```python
from build123d import *

# Parameters (mm, degrees)
F0_W      = 117
F0_H      = 85
F1_DEPTH  = 3.5
F2_R      = 4.5
F3_DEPTH  = 25
F4_R      = 30
F5_DEPTH  = 1
F7_R      = 25
F8_DEPTH  = 2
F9_R      = 20
F10_DEPTH = 2
F11_R     = 1
F12_R     = 10
F13_DEPTH = 25


# Not quite as in the source:
# - a fillet or chamfer that OpenCascade refuses, or shapes differently, is made with other operations: its cross-section is extruded or revolved along the edge and cut away or added


with BuildPart() as f1:
    # F0 (on Top) → F1 (new body)
    with BuildSketch(Plane.XY):
        Rectangle(F0_W, F0_H)
    extrude(amount=F1_DEPTH)

    # F2 (on face) → F3 (cut)
    with BuildSketch(Plane.XY.offset(3.5)):
        with Locations((40, 30)):
            Circle(F2_R)
        with Locations((-40, 30)):
            Circle(F2_R)
        with Locations((-40, -30)):
            Circle(F2_R)
        with Locations((40, -30)):
            Circle(F2_R)
    extrude(amount=-F3_DEPTH, mode=Mode.SUBTRACT)

    # F4 (on face) → F5 (join)
    with BuildSketch(Plane.XY.offset(3.5)):
        Circle(F4_R)
    extrude(amount=F5_DEPTH)

    # F6: fillet of radius 5 on 1 edges, made by hand

    # F6_s1 → F6_t2 (revolve, cut)
    with BuildSketch(Plane.XZ):
        with BuildLine():
            ThreePointArc((30, 3.5), (28.5811388301, 4.2434164903), (27, 4.5))
            Line((27, 4.5), (30, 4.5))
            Line((30, 4.5), (30, 3.5))
        make_face()
    revolve(axis=Axis((0, 0, 4.5), (0, 0, 1)), mode=Mode.SUBTRACT)

    # F7 (on face) → F8 (cut)
    with BuildSketch(Plane.XY.offset(4.5)):
        Circle(F7_R)
    extrude(amount=-F8_DEPTH, mode=Mode.SUBTRACT)

    # F9 (on face) → F10 (join)
    with BuildSketch(Plane.XY.offset(2.5)):
        Circle(F9_R)
    extrude(amount=F10_DEPTH)

    # F11
    f11_edges = [f1.edges().sort_by_distance(p)[0] for p in [
        (-20, 0, 4.5),
    ]]
    fillet(f11_edges, radius=F11_R)

    # F12 (on face) → F13 (cut)
    with BuildSketch(Plane.XY.offset(4.5)):
        Circle(F12_R)
    extrude(amount=-F13_DEPTH, mode=Mode.SUBTRACT)


solid = f1.part
```
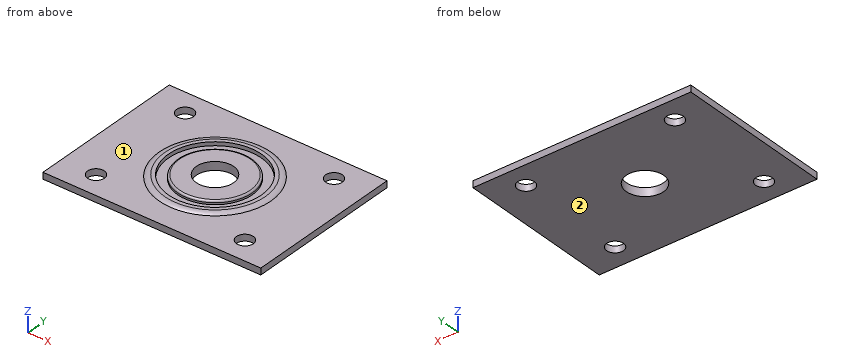
Geometry: final body of the model. Coordinates: model frame, mm. Face numbers are marked on the shaded views. Round coordinates to 2 decimals unless told otherwise and drop trailing zeros. Order: outer loops, then holes, each group sorted by start corner. A loop starts at its lowest first (then second) coordinate and runs counter-clockwise, first axis right, second up. Notation, with made-up numbers: (-4, 55.25) -> (30, 55.25) arc R26 cw to (30, 85.25) -> close; hole circle Ø7 at (-33, 56). An arc over 180 degrees is marked (long way). Use CSV: the item, a comma, the result in double quotes. Start each with the question number.
1) Section B-B (y = 0). Return the cut outline in (x, z), and give its area (3 significant figures).
2) Section D-D (x = 38.5). Return the cut outline in (y, z).
3) Section C-C (z = 1.25). Return the cut outline in (x, y), and give its area (3 significant figures).
4) First-contact query: pin 1 Ø3 at (x, y) = (35.5, 17.5) entering from +Z; pin 2 Ø2 at (x, y) = (-13.5, -18) entering from +Z. Flat tips, straight axial feed; report the tip coordinate or a pass-through.
5) Section A-A (x = -40). Return the cut outline in (y, z).
6) Material intervals for line 1 along Y through (x, z) = (40, 2.25); line 2 along X through (y, z) = (11, 3.45); line 3 along Y through (x, z) = (0, 3.85), sorted ascending. Write a range as from..to.
7) Draft query along Z for the marked faces 1 and 2. Return one class per face: +Z half, -Z half, draft (parallel to the pull), parting line (faces both ways), or undercut.
Returned:
1,outline,"(-58.5, 0) -> (-10, 0) -> (-10, 4.5) -> (-19, 4.5) arc R1 ccw to (-20, 3.5) -> (-20, 2.5) -> (-25, 2.5) -> (-25, 4.5) -> (-27, 4.5) arc R5 ccw to (-30, 3.5) -> (-58.5, 3.5) -> close; (10, 0) -> (58.5, 0) -> (58.5, 3.5) -> (30, 3.5) arc R5 ccw to (27, 4.5) -> (25, 4.5) -> (25, 2.5) -> (20, 2.5) -> (20, 3.5) arc R1 ccw to (19, 4.5) -> (10, 4.5) -> close"
1,area,"357 mm²"
2,outline,"(-42.5, 0) -> (-34.24, 0) -> (-34.24, 3.5) -> (-42.5, 3.5) -> close; (-25.76, 0) -> (25.76, 0) -> (25.76, 3.5) -> (-25.76, 3.5) -> close; (34.24, 0) -> (42.5, 0) -> (42.5, 3.5) -> (34.24, 3.5) -> close"
3,outline,"(-58.5, -42.5) -> (58.5, -42.5) -> (58.5, 42.5) -> (-58.5, 42.5) -> close; hole circle Ø9 at (-40, -30); hole circle Ø9 at (-40, 30); hole circle Ø20 at (0, 0); hole circle Ø9 at (40, -30); hole circle Ø9 at (40, 30)"
3,area,"9,380 mm²"
4,pin 1,"stops at z = 3.5"
4,pin 2,"stops at z = 2.5"
5,outline,"(-42.5, 0) -> (-34.5, 0) -> (-34.5, 3.5) -> (-42.5, 3.5) -> close; (-25.5, 0) -> (25.5, 0) -> (25.5, 3.5) -> (-25.5, 3.5) -> close; (34.5, 0) -> (42.5, 0) -> (42.5, 3.5) -> (34.5, 3.5) -> close"
6,line 1,"y = -42.5..-34.5, -25.5..25.5, 34.5..42.5"
6,line 2,"x = -58.5..-22.45, -16.7..16.7, 22.45..58.5"
6,line 3,"y = -29.47..-25, -19.94..-10, 10..19.94, 25..29.47"
7,face 1,"+Z half"
7,face 2,"-Z half"
